Job drawing, mm, ordinate dimensions from the low corner. One solid piece. A direction names the side the tool comes from. Give positions to 0.01 mm unless a question says otherwise; leave off trailing zeros. Loops run counter-clockwise (first coordinate to the right, second up) from the corner with the lowest first, then second, coordinate; pieces in that order, holes last. Notation, with made-up numbers: M 44.5,4.5 L 91.5,4.5 A13 ccw 91.5,17.5 Z; hole C 69.25,13 d10. An arc over 180 degrees is marked long. One line per question, with ' | ' between items.
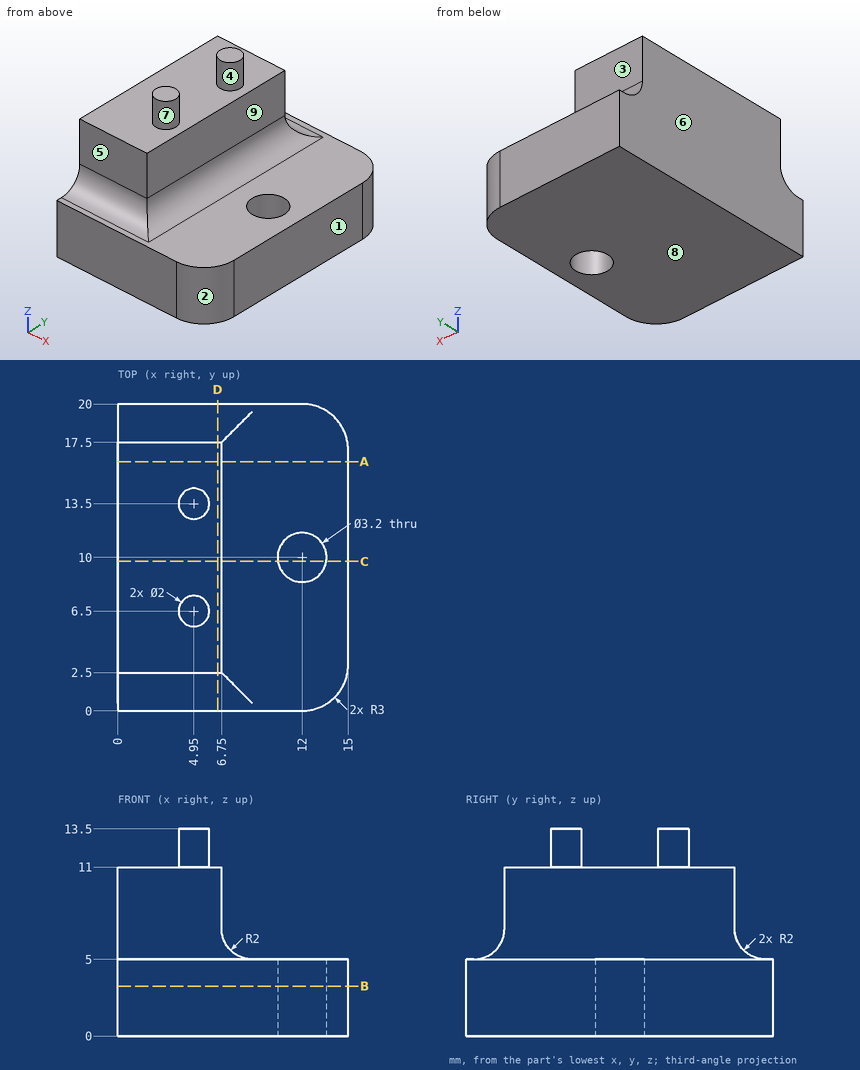
Item 1: Saw through at B-B on z = 3.25. Give the cut face in (x, y).
Conclusion:
outline: M 0,0 L 12,0 A3 ccw 15,3 L 15,17 A3 ccw 12,20 L 0,20 Z; hole C 12,10 d3.2
Item 2: Mould opens along Y. For the marked faces 1, 2, 3 and 4 say: pulls with the +Y half, pulls with the -Y half, needs draft (parallel to the pull), parting line crosses it, or undercut.
Conclusion:
face 1: needs draft | face 2: pulls with the -Y half | face 3: pulls with the +Y half | face 4: undercut
Item 3: Saw through at D-D on x = 6.5. Give the cut face in (y, z).
Conclusion:
outline: M 0,0 L 20,0 L 20,5 L 19.5,5 A2 cw 17.5,7 L 17.5,11 L 2.5,11 L 2.5,7 A2 cw 0.5,5 L 0,5 Z
Item 4: Saw through at A-A on y = 16.25. Give the cut face in (x, z), and give its area (3 significant figures).
Conclusion:
outline: M 0,0 L 15,0 L 15,5 L 8.75,5 A2 cw 6.75,7 L 6.75,11 L 0,11 Z | area: 116 mm²
Item 5: Drill centre lines: line 1 along Y through (x, z) = (12, 2); line 2 along Z through (x, y) = (3.25, 7.75); line 3 along Z through (x, y) = (11.75, 8). Where is each one in solid material? Low to high. Write a range as [from, to].
Conclusion:
line 1: [0, 8.4], [11.6, 20] | line 2: [0, 11] | line 3: [0, 5]
Item 6: 3-axis set-ups, long thin cutter, end or side, ignore diameter. For the marked faces 5, 6, 7, 8 and 9: which of +Z, -Z, +X, -X, +Y, -Y reach the whole face in a straight line?
Conclusion:
face 5: +Z, +X, -X, -Y | face 6: +Z, -Z, -X, +Y, -Y | face 7: +Z | face 8: -Z, +X, -X, +Y, -Y | face 9: +Z, +X, +Y, -Y
Item 7: Drop flat-ended pins along their axis: P1, Ø4, axis at x = 12, y = 10, coming from the +Z side; P2, Ø3, axis at x = 4.5, z = 9, coming from the -Y side; P3, Ø3, axis at x = 2.5, z = 9.5, coming from the +Y side. Give the stop position or say it passes through.
Conclusion:
P1: z = 5 | P2: y = 2.5 | P3: y = 17.5
Item 8: Saw through at C-C on y = 9.75. Give the cut face in (x, z).
Conclusion:
outline: M 0,0 L 10.42,0 L 10.42,5 L 8.75,5 A2 cw 6.75,7 L 6.75,11 L 0,11 Z; M 13.58,0 L 15,0 L 15,5 L 13.58,5 Z
